from build123d import *

# Parameters (mm, degrees)
SKETCH_1_W             = 64
SKETCH_1_H             = 16
EXTRUDE_1_DEPTH        = 20
SKETCH_3_R             = 2.125
CUT_EXTRUDE_1_DEPTH    = 28
SKETCH_4_W             = 36
SKETCH_4_H             = 10
CUT_EXTRUDE_2_DEPTH    = 20
SKETCH_5_W             = 64
SKETCH_5_H             = 10.5
CUT_EXTRUDE_3_DEPTH    = 10
HOLE_WIZARD_M5_1_D     = 4.2
HOLE_WIZARD_M5_1_DEPTH = 12.4
HOLE_WIZARD_M5_1_TIP   = 1.2618073
FILLET_1_R             = 3
FILLET_2_R             = 3
SKETCH_7_W             = 45
SKETCH_7_H             = 10.5
CUT_EXTRUDE_4_DEPTH    = 10
FILLET_3_R             = 3
FILLET_4_R             = 1


with BuildPart() as part:
    # 草图1 → 凸台-拉伸1 (new body)
    with BuildSketch(Plane(origin=(0, 0, 0), x_dir=(1, 0, 0), z_dir=(0, 1, 0))):
        Rectangle(SKETCH_1_W, SKETCH_1_H)
    extrude(amount=EXTRUDE_1_DEPTH)

    # 草图3 → 切除-拉伸1 (cut)
    with BuildSketch(Plane.XY.offset(8)):
        with Locations((-25, 4)):
            Circle(SKETCH_3_R)
        with Locations((25, 4)):
            Circle(SKETCH_3_R)
    extrude(amount=-CUT_EXTRUDE_1_DEPTH, mode=Mode.SUBTRACT)

    # 草图4 → 切除-拉伸2 (cut)
    with BuildSketch(Plane.XY.offset(8)):
        with Locations((0, 5)):
            Rectangle(SKETCH_4_W, SKETCH_4_H)
    extrude(amount=-CUT_EXTRUDE_2_DEPTH, mode=Mode.SUBTRACT)

    # 草图5 → 切除-拉伸3 (cut)
    with BuildSketch(Plane.XZ):
        Rectangle(SKETCH_5_W, SKETCH_5_H)
    extrude(amount=-CUT_EXTRUDE_3_DEPTH, mode=Mode.SUBTRACT)

    # M5 螺纹孔1
    with Locations(Plane(origin=(27.223611076, 20, 0), x_dir=(0, 0, 1), z_dir=(0, 1, 0))):
        with Locations((0, 0), (0, -54.447222152)):
            Hole(HOLE_WIZARD_M5_1_D / 2, depth=HOLE_WIZARD_M5_1_DEPTH)
            with Locations((0, 0, -(HOLE_WIZARD_M5_1_DEPTH + HOLE_WIZARD_M5_1_TIP / 2))):  # 118° drill point
                Cone(0, HOLE_WIZARD_M5_1_D / 2, HOLE_WIZARD_M5_1_TIP, mode=Mode.SUBTRACT)

    # 圆角1
    fillet_1_edges = [part.edges().sort_by_distance(p)[0] for p in [
        (-18, 0, -6.625),
        (18, 0, 6.625),
        (-18, 0, 6.625),
        (18, 0, -6.625),
        (-32, 0, 6.625),
        (-32, 0, -6.625),
        (32, 0, -6.625),
        (32, 0, 6.625),
    ]]
    fillet(fillet_1_edges, radius=FILLET_1_R)

    # 圆角2
    fillet_2_edges = [part.edges().sort_by_distance(p)[0] for p in [
        (-18, 10, -6.625),
        (18, 10, -6.625),
        (-18, 10, 6.625),
        (18, 10, 6.625),
    ]]
    fillet(fillet_2_edges, radius=FILLET_2_R)

    # 草图7 → 切除-拉伸4 (cut)
    with BuildSketch(Plane(origin=(0, 20, 0), x_dir=(1, 0, 0), z_dir=(0, 1, 0))):
        Rectangle(SKETCH_7_W, SKETCH_7_H)
    extrude(amount=-CUT_EXTRUDE_4_DEPTH, mode=Mode.SUBTRACT)

    # 圆角3
    fillet_3_edges = [part.edges().sort_by_distance(p)[0] for p in [
        (22.5, 15, -5.25),
        (22.5, 15, 5.25),
        (-22.5, 15, 5.25),
        (-22.5, 15, -5.25),
    ]]
    fillet(fillet_3_edges, radius=FILLET_3_R)

    # 圆角4
    fillet_4_edges = [part.edges().sort_by_distance(p)[0] for p in [
        (31.121320344, 0.878679656, -8),
        (25, 0, 8),
        (18, 5, 8),
        (-25, 0, 8),
        (-18.878679656, 0.878679656, 8),
        (-31.121320344, 0.878679656, 8),
        (18.878679656, 0.878679656, 8),
        (31.121320344, 0.878679656, 8),
        (-32, 20, 0),
        (0, 10, -8),
        (0, 10, 8),
        (-18, 5, -8),
        (-18, 5, 8),
        (17.121320344, 9.121320344, -8),
        (17.121320344, 9.121320344, 8),
        (-17.121320344, 9.121320344, -8),
        (-17.121320344, 9.121320344, 8),
        (0, 20, 8),
        (32, 20, 0),
        (32, 11.5, 8),
        (-32, 11.5, 8),
        (-32, 11.5, -8),
        (32, 11.5, -8),
        (0, 20, -8),
        (25, 0, -8),
        (18, 5, -8),
        (-25, 0, -8),
        (-31.121320344, 0.878679656, -8),
        (-18.878679656, 0.878679656, -8),
        (18.878679656, 0.878679656, -8),
    ]]
    fillet(fillet_4_edges, radius=FILLET_4_R)


solid = part.part
Could you check a few things on this model? Use its own coordinates, in mm. A direction names the side the tool comes from. Round coordinates to 2 decimals unless told otherwise and drop trailing zeros. Write each loop counter-clockwise with the first axis right and the second up, starting at its lowest first coordinate (ties: lowest second). Pieces come first, ordered by that corner, then holes. Notation, with made-up numbers: (50.25, 10) - (99.25, 10) arc R15 ccw to (99.25, 18) - close; hole circle Ø1 at (-18.75, 4.5). An arc over 180 degrees is marked (long way). Put each result on its own line as item: value. Start each with the question number.
(1) I want a section at A-A, the plane x = 9.5. Please give me the cut outline in (y, z).
(2) I want a section at C-C, the plane y = 4. Give the number of separate pieces and of enclosed holes in the cut face, plus the area to 3 significant figures.
(3) I want a section at B-B, the plane z = 0. Please give me the cut outline in (x, y), plus the area to 3 significant figures.
(4) I want a section at D-D, the plane z = 3.75. Please give me the cut outline in (x, y), plus the area to 3 significant figures.
(5) Will these pins go through, and if not, where does the flat tip stop? pin 1 (8 mm diameter, centred on x = 13, z = 6, fed in from -Y); pin 2 (1.9 mm diameter, centred on x = -7, z = 6.5, fed in from -Y); pin 3 (4 mm diameter, centred on y = 2.5, z = 2, fed in from +X).
(6) I need wall thicknesses on probe 1 along X at (y, z) = (13.25, 0); probe 2 along Z at (x, y) = (9, 12.5); probe 3 along Y at (x, z) = (-25, -6.5) (3 decimals). Which ranges of each line are inside material? Lowest first, please.
(7) For faces 1 (the cylindrical face through (-18.9, 0.86, -6.14)), 2 (the flat face through (-32, 13, 0)), 3 (the flat face through (-27.2, 10, 2.4)), 4 (the cylindrical face through (-21.6, 14.93, 4.39)), which set-ups out of +Z, -Z, +X, -X, +Y, -Y let a thin tool reach every point of the face, with its end or its side?
(8) Thinking about a two-plate mould opening in Z: for faces 5 (the flat face through (27.1, 10, 2.4)), 6 (the flat face through (0, 10, -6)), 7 (the cylindrical face through (21.6, 14.93, 4.39)), which applies, released by +Z, released by -Z, zero draft, split by the parting line, or undercut?
Here are the results:
1. outline: (10, -7) arc R1 ccw to (11, -8) - (19, -8) arc R1 ccw to (20, -7) - (20, -5.25) - (10, -5.25) - close; (10, 5.25) - (20, 5.25) - (20, 7) arc R1 ccw to (19, 8) - (11, 8) arc R1 ccw to (10, 7) - close
2. separate pieces: 8
2. enclosed holes: 0
2. area: 106 mm^2
3. outline: (-32, 10) - (-29.32, 10) - (-29.32, 20) - (-31, 20) arc R1 ccw to (-32, 19) - close; (-25.12, 10) - (-22.5, 10) - (-22.5, 20) - (-25.12, 20) - close; (22.5, 10) - (25.12, 10) - (25.12, 20) - (22.5, 20) - close; (29.32, 10) - (32, 10) - (32, 19) arc R1 ccw to (31, 20) - (29.32, 20) - close
3. area: 106 mm^2
4. outline: (-32, 10) - (-22.1, 10) - (-22.1, 20) - (-31, 20) arc R1 ccw to (-32, 19) - close; (22.1, 10) - (32, 10) - (32, 19) arc R1 ccw to (31, 20) - (22.1, 20) - close
4. area: 198 mm^2
5. pin 1: stops at y = 9.24
5. pin 2: stops at y = 10
5. pin 3: passes through
6. probe 1: x = -32 to -29.32, -25.12 to -22.5, 22.5 to 25.12, 29.32 to 32
6. probe 2: z = -8 to -5.25, 5.25 to 8
6. probe 3: y = 0 to 1.875, 6.125 to 20
7. face 1: +Z, -Z, -Y
7. face 2: +Z, -Z, -X, +Y, -Y
7. face 3: +X, -X, -Y
7. face 4: +Y, -Y
8. face 5: undercut
8. face 6: zero draft
8. face 7: undercut
